Design review of the part built by this model. Coordinates are the model's own, in mm. Coordinates: 2 decimals unless noted, no trailing zeros. Loops run counter-clockwise (first coordinate to the right, second up) from the corner with the lowest first, then second, coordinate; pieces in that order, holes last. Notation, with made-up numbers: (53.5, 74.5) -> (88.5, 74.5) arc R10 ccw to (88.5, 93.5) -> close; hole circle Ø2 at (68.25, 66.25). An arc over 180 degrees is marked (long way). Answer as a JSON object with one key per item and string values.
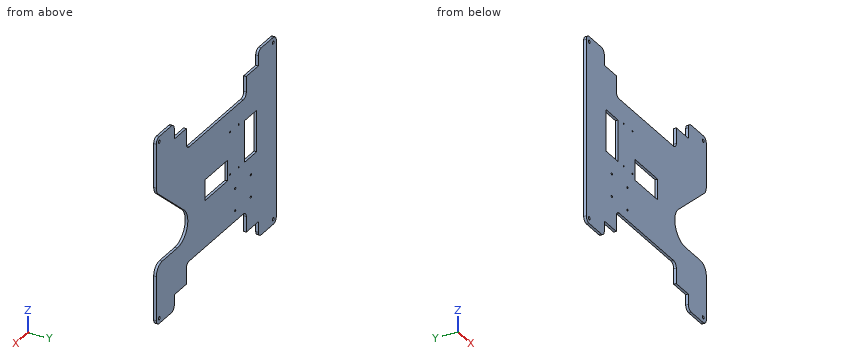
```python
from build123d import *

# Parameters (mm, degrees)
SKETCH_4_R                = 15
EXTRUDE_1_DEPTH           = 5
SKETCH_6_R                = 1.5
SKETCH_6_R_2              = 2
SKETCH_6_R_3              = 1.6
SKETCH_6_R_4              = 1.75
CUT_EXTRUDE_2_DEPTH       = 5
SKETCH_8_R                = 3
CUT_EXTRUDE_4_DEPTH       = 10
FILLET_1_R                = 10
CUT_EXTRUDE_24_DEPTH      = 270.118932816
CUT_EXTRUDE_24_DEPTH_BACK = 270.118932816
SKETCH_23_W               = 75
SKETCH_23_H               = 40
SKETCH_23_W_2             = 40
SKETCH_23_H_2             = 80
CUT_EXTRUDE_26_DEPTH      = 270.118932816
FILLET_2_R                = 20


with BuildPart() as part:
    # 草圖4 → 伸長1 (new body)
    with BuildSketch(Plane(origin=(0, 0, 0), x_dir=(1, 0, 0), z_dir=(0, 1, 0))):
        Polygon((-200, 180), (-140, 180), (-140, 150), (-100, 150), (-100, 110), (100, 110), (100, 150), (140, 150), (140, 180), (200, 180), (200, -180), (140, -180), (140, -150), (100, -150), (100, -110), (-100, -110), (-100, -150), (-140, -150), (-140, -180), (-200, -180), align=None)
        with Locations(Location((0, 0, 0), (0, 0, 270))):
            Circle(SKETCH_4_R, mode=Mode.SUBTRACT)
    extrude(amount=EXTRUDE_1_DEPTH)

    # 草圖6 → 伸長2 (cut)
    with BuildSketch(Plane(origin=(0, 5, 0), x_dir=(-1, 0, 0), z_dir=(0, 1, 0))):
        with Locations(Location((75, -12, 0), (0, 0, 90))):
            Circle(SKETCH_6_R)
        with Locations(Location((46, -12, 0), (0, 0, 90))):
            Circle(SKETCH_6_R)
        with Locations(Location((46, 70, 0), (0, 0, 90))):
            Circle(SKETCH_6_R)
        with Locations(Location((75, 70, 0), (0, 0, 90))):
            Circle(SKETCH_6_R)
        with Locations(Location((63, -90, 0), (0, 0, 90))):
            Circle(SKETCH_6_R_2)
        with Locations(Location((115, -90, 0), (0, 0, 90))):
            Circle(SKETCH_6_R_2)
        with Locations(Location((115, -47, 0), (0, 0, 90))):
            Circle(SKETCH_6_R_2)
        with Locations(Location((63, -47, 0), (0, 0, 90))):
            Circle(SKETCH_6_R_2)
        with Locations(Location((130, -10, 0), (0, 0, 90))):
            Circle(SKETCH_6_R_3)
        with Locations(Location((130, 65, 0), (0, 0, 90))):
            Circle(SKETCH_6_R_3)
        with Locations(Location((99, 65, 0), (0, 0, 90))):
            Circle(SKETCH_6_R_3)
        with Locations(Location((99, -10, 0), (0, 0, 90))):
            Circle(SKETCH_6_R_3)
        with Locations(Location((33, 16.5, 0), (0, 0, 90))):
            Circle(SKETCH_6_R_4)
        with Locations(Location((33, -16.5, 0), (0, 0, 90))):
            Circle(SKETCH_6_R_4)
        with Locations(Location((-33, -16.5, 0), (0, 0, 90))):
            Circle(SKETCH_6_R_4)
        with Locations(Location((-33, 16.5, 0), (0, 0, 90))):
            Circle(SKETCH_6_R_4)
    extrude(amount=-CUT_EXTRUDE_2_DEPTH, mode=Mode.SUBTRACT)

    # 草圖8 → 伸長4 (cut)
    with BuildSketch(Plane(origin=(0, 5, 0), x_dir=(1, 0, 0), z_dir=(0, 1, 0))):
        with Locations(Location((190, 170, 0), (0, 0, 270))):
            Circle(SKETCH_8_R)
        with Locations(Location((-190, 170, 0), (0, 0, 270))):
            Circle(SKETCH_8_R)
        with Locations(Location((-190, -170, 0), (0, 0, 270))):
            Circle(SKETCH_8_R)
        with Locations(Location((190, -170, 0), (0, 0, 270))):
            Circle(SKETCH_8_R)
    extrude(amount=-CUT_EXTRUDE_4_DEPTH, mode=Mode.SUBTRACT)

    # 圓角1
    fillet_1_edges = [part.edges().sort_by_distance(p)[0] for p in [
        (-200, 2.5, -180),
        (-140, 2.5, -180),
        (-100, 2.5, -110),
        (100, 2.5, -110),
        (140, 2.5, -180),
        (200, 2.5, -180),
        (200, 2.5, 180),
        (140, 2.5, 180),
        (100, 2.5, 110),
        (-100, 2.5, 110),
        (-140, 2.5, 180),
        (-200, 2.5, 180),
    ]]
    fillet(fillet_1_edges, radius=FILLET_1_R)

    # 草圖21 → 伸長24 (cut, two sides: drawn at the far end of the back side and taken through both)
    with BuildSketch(Plane(origin=(0, 5, 0), x_dir=(1, 0, 0), z_dir=(0, 1, 0)).offset(-CUT_EXTRUDE_24_DEPTH_BACK)):
        with BuildLine():
            Line((1160.368223513, 65), (200, 65))
            Line((200, 65), (130, 65))
            ThreePointArc((130, 65), (97.189752759, 42.185551936), (107.153658755, 3.485010057))
            Line((107.153658755, 3.485010057), (200, -76.514989943))
            Line((200, -76.514989943), (927.547251098, -703.397851531))
            Line((927.547251098, -703.397851531), (2765.756739288, -1260.366770288))
            Line((2765.756739288, -1260.366770288), (2998.577711703, -491.968918756))
            Line((2998.577711703, -491.968918756), (1160.368223513, 65))
        make_face()
    extrude(amount=CUT_EXTRUDE_24_DEPTH + CUT_EXTRUDE_24_DEPTH_BACK, mode=Mode.SUBTRACT)

    # 草圖23 → 伸長26 (cut, through all)
    with BuildSketch(Plane(origin=(0, 5, 0), x_dir=(1, 0, 0), z_dir=(0, 1, 0))):
        Rectangle(SKETCH_23_W, SKETCH_23_H)
        with Locations((-114.5, -27.5)):
            Rectangle(SKETCH_23_W_2, SKETCH_23_H_2)
    extrude(amount=-CUT_EXTRUDE_26_DEPTH, mode=Mode.SUBTRACT)

    # 圓角2
    fillet_2_edges = [part.edges().sort_by_distance(p)[0] for p in [
        (200, 2.5, 76.514989943),
        (200, 2.5, -65),
    ]]
    fillet(fillet_2_edges, radius=FILLET_2_R)


solid = part.part
```
1) Add section C-C, the plane x = 58.5. Give the boundary of the cut face in (y, z).
Completed:
{"outline": "(0, -110) -> (5, -110) -> (5, 110) -> (0, 110) -> close"}
2) Wall thickness on probe 1 along X at (y, z) = (2.45, -12); probe 2 along Z at (x, y) = (-75, 3.05); probe 3 along X at (y, z) = (3.6, 170): over which ranges is each line inside the solid? List them lowest first.
Completed:
{"probe 1": "-200 to -134.5, -94.5 to -76.5, -73.5 to -47.5, -44.5 to -37.5, 37.5 to 99.98", "probe 2": "-110 to -13.5, -10.5 to 68.5, 71.5 to 110", "probe 3": "-200 to -193, -187 to -140, 140 to 187, 193 to 200"}
3) Add section B-B, the plane z = 51. Give the boundary of the cut face in (x, y), and give its area (3 significant figures).
Completed:
{"outline": "(-200, 0) -> (-134.5, 0) -> (-134.5, 5) -> (-200, 5) -> close; (-94.5, 0) -> (170.39, 0) -> (170.39, 5) -> (-94.5, 5) -> close", "area": "1,650 mm²"}
4) Add section A-A, the plane x = -123.5. Give the boundary of the cut face in (y, z).
Completed:
{"outline": "(0, -150) -> (5, -150) -> (5, -12.5) -> (0, -12.5) -> close; (0, 67.5) -> (5, 67.5) -> (5, 150) -> (0, 150) -> close"}
5) Clearance check with flat-ended pins moving along their axes: pin 1 Ø1.5 at (x, y) = (-116, 2.5) entering from -Z; pin 2 Ø4 at (x, z) = (-46, 70) entering from -Y; pin 3 Ø2 at (x, y) = (-97.5, 0.5) entering from -Z; pin 4 Ø5 at (x, z) = (190, 170) entering from -Y. State where each tip first meets the part, or that it passes through.
Completed:
{"pin 1": "z = -150", "pin 2": "y = 0", "pin 3": "z = -114.73", "pin 4": "through"}
6) Add section D-D, the plane y = 1.9. Count the separate pieces of the cut face and the enclosed holes in it, and give its area (3 significant figures).
Completed:
{"separate pieces": "1", "enclosed holes": "14", "area": "94,800 mm²"}
